Can you work these out from the model? Positions are in its coordinate system, mm. Face numbers are marked on the shaded views. Give positions to 0.01 mm unless a question says otherwise; leave off trailing zeros. Order: outer loops, then holes, each group sorted by start corner. A loop starts at its lowest first (then second) coordinate and runs counter-clockwise, first axis right, second up. Notation, with made-up numbers: (51, 86) -> (80, 86) arc R22 cw to (80, 105) -> close; hole circle Ø6 at (3.5, -26.75). An arc over 180 degrees is marked (long way). Answer as a JSON object with one key per item and string values.
```python
from build123d import *

# Parameters (mm, degrees)
SKIZZE1_R                       = 300
AUFSATZ_LINEAR_AUSTRAGEN1_DEPTH = 300
SKIZZE2_R                       = 20
SCHNITT_LINEAR_AUSTRAGEN1_DEPTH = 300
SKIZZE3_R                       = 200
SKIZZE3_R_2                     = 60
SCHNITT_LINEAR_AUSTRAGEN2_DEPTH = 20


with BuildPart() as part:
    # Skizze1 → Aufsatz-Linear austragen1 (new body)
    with BuildSketch(Plane.XY):
        Circle(SKIZZE1_R)
    extrude(amount=AUFSATZ_LINEAR_AUSTRAGEN1_DEPTH)

    # Skizze2 → Schnitt-Linear austragen1 (cut)
    with BuildSketch(Plane.XY.offset(300)):
        Circle(SKIZZE2_R)
    extrude(amount=-SCHNITT_LINEAR_AUSTRAGEN1_DEPTH, mode=Mode.SUBTRACT)

    # Skizze3 → Schnitt-Linear austragen2 (cut)
    with BuildSketch(Plane.XY.offset(300)):
        Circle(SKIZZE3_R)
        Circle(SKIZZE3_R_2, mode=Mode.SUBTRACT)
    extrude(amount=-SCHNITT_LINEAR_AUSTRAGEN2_DEPTH, mode=Mode.SUBTRACT)


solid = part.part
```
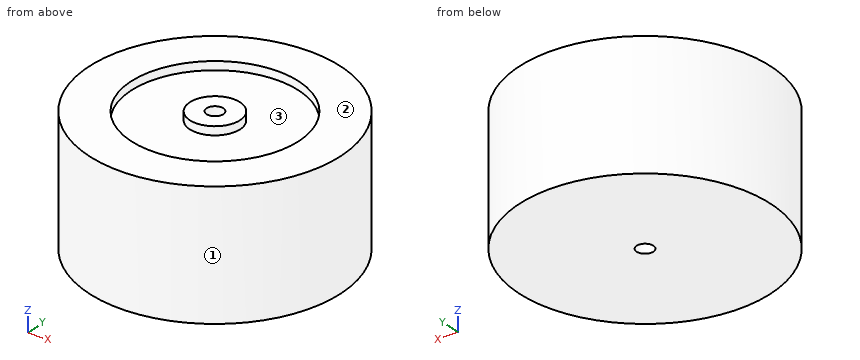
1. Will these pins go through, and if not, where does the flat tip stop? pin 1 Ø6 at (x, y) = (159, 137) entering from -Z; pin 2 Ø2 at (x, z) = (54, 72) entering from -Y; pin 3 Ø12 at (y, z) = (-94, 207) entering from +X; pin 4 Ø5 at (x, z) = (-162.5, 209) entering from +Y.
Worked answers:
{"pin 1": "z = 0", "pin 2": "y = -295.28", "pin 3": "x = 286.8", "pin 4": "y = 253.77"}
2. If we section it at C-C on z = 270: Please give me the cut outline in (x, y), then the cut area to 3 significant figures.
Worked answers:
{"outline": "circle Ø600 at (0, 0); hole circle Ø40 at (0, 0)", "area": "281,000 mm²"}
3. If we section it at D-D on x = 117: Please give me the cut outline in (y, z).
Worked answers:
{"outline": "(-276.24, 0) -> (276.24, 0) -> (276.24, 300) -> (162.21, 300) -> (162.21, 280) -> (-162.21, 280) -> (-162.21, 300) -> (-276.24, 300) -> close"}
4. If we section it at A-A on x = 0: Please give me the cut outline in (y, z), then the cut area to 3 significant figures.
Worked answers:
{"outline": "(-300, 0) -> (-20, 0) -> (-20, 300) -> (-60, 300) -> (-60, 280) -> (-200, 280) -> (-200, 300) -> (-300, 300) -> close; (20, 0) -> (300, 0) -> (300, 300) -> (200, 300) -> (200, 280) -> (60, 280) -> (60, 300) -> (20, 300) -> close", "area": "162,000 mm²"}
5. Please list where these lines run through material, in increasing order: L1, parallel to Y at x = 0, z = 292.25; L2, parallel to Y at x = 0, z = 135; L3, parallel to Z at x = 28.5, y = -57.
Worked answers:
{"L1": "-300 to -200, -60 to -20, 20 to 60, 200 to 300", "L2": "-300 to -20, 20 to 300", "L3": "0 to 280"}
6. If we mould it in two halves opening along Y, with no side actions, what happens to the marked faces 1, 2 and 3? For each: +Y half, -Y half, draft (parallel to the pull), parting line (faces both ways), or undercut.
Worked answers:
{"face 1": "parting line", "face 2": "draft", "face 3": "undercut"}
